Verification items for the finished model (mm, model axes). A direction names the side the tool comes from. Round coordinates to 2 decimals unless told otherwise and drop trailing zeros. Write each loop counter-clockwise with the first axis right and the second up, starting at its lowest first coordinate (ties: lowest second). Pieces come first, ordered by that corner, then holes. Notation, with made-up numbers: M 50.5,-21.5 L 83.5,-21.5 A25 ccw 83.5,6.5 Z; hole C -9.75,56.25 d4. An arc over 180 degrees is marked long. One line per question, with ' | ' between items. Start each with the question number.
Q1. Tool access check on faces 5 (the face through (8, 13.5, 14)), 6 (the face through (5.2, 25, -0.2)). Record the directions out of +Z, -Z, +X, -X, +Y, -Y that give a thin tool (end or side, any length) a straight path to the whole face; none if there is none.
Q2. Cross-section at B-B (x = 0). Record the boundary of the cut face in (y, z) (3 decimals), then the cut area to 3 significant figures.
Q3. Cross-section at D-D (x = 11.5). Record the boundary of the cut face in (y, z).
Q4. Release check for a two-part mould opening along Y. For faces 1 (the face through (15.18, 7.42, 4.78)), 2 (the face through (-11.99, 19.93, -0.53)), 3 (the face through (-12, 15, 4)), 4 (the face through (8, 1.5, -14)) record: released by +Y, released by -Y, zero draft, split by the parting line, or undercut.
Q5. Cross-section at A-A (z = 0). Record the boundary of the cut face in (x, y) (3 decimals).
Q6. Gauge pin test, flat ends, axial feed: pin 1 (10 mm diameter, centred on x = 12.5, y = 6.5, fed in from +Z); pin 2 (4 mm diameter, centred on y = 12, z = 8, fed in from +X); pin 3 (3 mm diameter, centred on x = -2, y = 6.5, fed in from +Z). Record the tip position at first contact, or that the pin passes through.
Q7. Thickness scan on line 1 along Z through (x, y) = (0, 17.5); line 2 along X through (y, z) = (11.25, 0) (3 decimals); line 3 along Y through (x, z) = (8.5, 14.5). Record the ranges inside material, lowest first. Write a range as from..to.
Q8. Cross-section at C-C (y = 11.5). Record the boundary of the cut face in (x, z) (3 decimals), then the cut area to 3 significant figures.
from build123d import *

# Parameters (mm, degrees)
SKETCH1_R           = 32.34
BOSS_EXTRUDE1_DEPTH = 15
SKETCH2_R           = 12
BOSS_EXTRUDE2_DEPTH = 10
SKETCH3_R           = 5
CUT_EXTRUDE1_DEPTH  = 26
SKETCH4_R           = 32.34
SKETCH4_R_2         = 15.915
CUT_EXTRUDE3_DEPTH  = 15
SKETCH5_R           = 17.5
SKETCH5_R_2         = 15.915
BOSS_EXTRUDE3_DEPTH = 1.5
SKETCH6_R           = 17.5
SKETCH6_R_2         = 15.915
BOSS_EXTRUDE4_DEPTH = 1.5


with BuildPart() as part:
    # Sketch1 → Boss-Extrude1 (new body)
    with BuildSketch(Plane(origin=(0, 0, 0), x_dir=(1, 0, 0), z_dir=(0, 1, 0))):
        Circle(SKETCH1_R)
    extrude(amount=BOSS_EXTRUDE1_DEPTH)

    # Sketch2 → Boss-Extrude2 (add)
    with BuildSketch(Plane(origin=(0, 15, 0), x_dir=(1, 0, 0), z_dir=(0, 1, 0))):
        Circle(SKETCH2_R)
    extrude(amount=BOSS_EXTRUDE2_DEPTH)

    # Sketch3 → Cut-Extrude1 (cut)
    with BuildSketch(Plane(origin=(0, 25, 0), x_dir=(1, 0, 0), z_dir=(0, 1, 0))):
        Circle(SKETCH3_R)
    extrude(amount=-CUT_EXTRUDE1_DEPTH, mode=Mode.SUBTRACT)

    # Sketch4 → Cut-Extrude3 (cut)
    with BuildSketch(Plane.XZ):
        Circle(SKETCH4_R)
        Circle(SKETCH4_R_2, mode=Mode.SUBTRACT)
    extrude(amount=-CUT_EXTRUDE3_DEPTH, mode=Mode.SUBTRACT)

    # Sketch5 → Boss-Extrude3 (add)
    with BuildSketch(Plane.XZ):
        Circle(SKETCH5_R)
        Circle(SKETCH5_R_2, mode=Mode.SUBTRACT)
    extrude(amount=-BOSS_EXTRUDE3_DEPTH)

    # Sketch6 → Boss-Extrude4 (add)
    with BuildSketch(Plane(origin=(0, 15, 0), x_dir=(1, 0, 0), z_dir=(0, 1, 0))):
        Circle(SKETCH6_R)
        Circle(SKETCH6_R_2, mode=Mode.SUBTRACT)
    extrude(amount=-BOSS_EXTRUDE4_DEPTH)


solid = part.part
Determined:
1) face 5: none | face 6: +Z, -Z, +X, -X, +Y
2) outline: M 0,-17.5 L 1.5,-17.5 L 1.5,-15.915 L 13.5,-15.915 L 13.5,-17.5 L 15,-17.5 L 15,-12 L 25,-12 L 25,-5 L 0,-5 Z; M 0,5 L 25,5 L 25,12 L 15,12 L 15,17.5 L 13.5,17.5 L 13.5,15.915 L 1.5,15.915 L 1.5,17.5 L 0,17.5 Z | area: 477 mm²
3) outline: M 0,-13.19 L 1.5,-13.19 L 1.5,-11 L 13.5,-11 L 13.5,-13.19 L 15,-13.19 L 15,-3.43 L 25,-3.43 L 25,3.43 L 15,3.43 L 15,13.19 L 13.5,13.19 L 13.5,11 L 1.5,11 L 1.5,13.19 L 0,13.19 Z
4) face 1: undercut | face 2: zero draft | face 3: released by +Y | face 4: undercut
5) outline: M -17.5,0 L -5,0 L -5,25 L -12,25 L -12,15 L -17.5,15 L -17.5,13.5 L -15.915,13.5 L -15.915,1.5 L -17.5,1.5 Z; M 5,0 L 17.5,0 L 17.5,1.5 L 15.915,1.5 L 15.915,13.5 L 17.5,13.5 L 17.5,15 L 12,15 L 12,25 L 5,25 Z
6) pin 1: stops at z = 14.04 | pin 2: stops at x = 16.18 | pin 3: stops at z = 15.91
7) line 1: z = -12..-5, 5..12 | line 2: x = -15.915..-5, 5..15.915 | line 3: y = 0..1.5, 13.5..15
8) outline: C 0,0 d31.83; hole C 0,0 d10 | area: 717 mm²
